Design review of the part built by this model. Coordinates are the model's own, in mm. A direction names the side the tool comes from. Give positions to 0.01 mm unless a question says otherwise; leave off trailing zeros. Order: outer loops, then holes, each group sorted by start corner. A loop starts at its lowest first (then second) coordinate and runs counter-clockwise, first axis right, second up. Notation, with made-up numbers: (26, 59.5) -> (50, 59.5) arc R22 cw to (50, 96.5) -> close; hole circle Ø11 at (71.25, 46.5). An arc over 180 degrees is marked (long way). Return JSON: item names as keys, results as strings.
```python
from build123d import *


with BuildPart() as part:
    # Эскиз1 → Повернуть1 (revolve)
    with BuildSketch(Plane.XY, mode=Mode.PRIVATE) as revolve_1_sk:
        with BuildLine():
            Line((0, 0), (0, 112))
            Line((0, 112), (2.6, 112))
            Line((2.6, 112), (3.9, 110.7))
            Line((3.9, 110.7), (3.9, 13.6))
            ThreePointArc((3.9, 13.6), (6.536038969, 7.236038969), (12.9, 4.6))
            Line((12.9, 4.6), (13.537009085, 4.6))
            Line((13.537009085, 4.6), (15.5, 1.2))
            Line((15.5, 1.2), (15.5, 0))
            Line((15.5, 0), (0, 0))
        make_face()
    revolve(revolve_1_sk.sketch.rotate(Axis((0, 0, 0), (0, 1, 0)), 90), axis=Axis((0, 0, 0), (0, 1, 0)))


solid = part.part
```
Item 1: Wall thickness on L1, parallel to Y at x = -10.5, z = -7.5; L2, parallel to X at y = 43, z = -1; L3, parallel to Y at x = 7, z = 0.5: over which ranges is each line inside the solid? List them lowest first. Write a range as [from, to].
Result set:
{"L1": "y = [0, 4.6]", "L2": "x = [-3.77, 3.77]", "L3": "y = [0, 6.79]"}
Item 2: Add section A-A (z = 0). Give the boundary of the cut face in (x, y), plus the area to 3 significant figures.
Result set:
{"outline": "(-15.5, 0) -> (15.5, 0) -> (15.5, 1.2) -> (13.54, 4.6) -> (12.9, 4.6) arc R9 cw to (3.9, 13.6) -> (3.9, 110.7) -> (2.6, 112) -> (-2.6, 112) -> (-3.9, 110.7) -> (-3.9, 13.6) arc R9 cw to (-12.9, 4.6) -> (-13.54, 4.6) -> (-15.5, 1.2) -> close", "area": "1,010 mm^2"}
Item 3: Machinability: for faces 1 (the face through (-2.64, 61.47, 2.87)), 2 (the face through (0, 0, 0)), which of the approach directions +Z, -Z, +X, -X, +Y, -Y give a long, thin tool a straight path to every point of the face, cutting with its end or side? Answer none if there is none.
Result set:
{"face 1": "+Y", "face 2": "+Z, -Z, +X, -X, -Y"}
Item 4: Add section B-B (x = 0). Give the boundary of the cut face in (y, z), plus the area to 3 significant figures.
Result set:
{"outline": "(0, -15.5) -> (1.2, -15.5) -> (4.6, -13.54) -> (4.6, -12.9) arc R9 cw to (13.6, -3.9) -> (110.7, -3.9) -> (112, -2.6) -> (112, 2.6) -> (110.7, 3.9) -> (13.6, 3.9) arc R9 cw to (4.6, 12.9) -> (4.6, 13.54) -> (1.2, 15.5) -> (0, 15.5) -> close", "area": "1,010 mm^2"}
Item 5: For pin 1 (2 mm diameter, centred on x = 6.5, y = 23.5, fed in from +Z); pin 2 (1 mm diameter, centred on x = 2, z = -8.5, fed in from +Y); pin 3 (4 mm diameter, centred on y = 72.5, z = -1, fed in from -X); pin 4 (1 mm diameter, centred on x = 0, z = 8, fed in from +Y), all flat-tipped, find the tip position at first contact; note any pin that passes through.
Result set:
{"pin 1": "passes through", "pin 2": "stops at y = 5.91", "pin 3": "stops at x = -3.9", "pin 4": "stops at y = 6.4"}
